Work out the finished part from the listing and answer in its coordinate system (mm). A direction names the side the tool comes from. Give positions to 0.01 mm unless a question says otherwise; leave off trailing zeros. Order: outer loops, then holes, each group sorted by start corner. A loop starts at its lowest first (then second) coordinate and runs counter-clockwise, first axis right, second up. Notation, with made-up numbers: (20.25, -26.5) -> (27.25, -26.5) arc R34 ccw to (27.25, 10.5) -> close; hole circle Ø6 at (52, -12.5). An arc over 180 degrees is marked (long way). Use a Markdown table: item, result. Add a question column.
```python
from build123d import *

# Parameters (mm, degrees)
BOSS_EXTRUDE1_DEPTH         = 10
CHAMFER1_SIZE               = 10
F_1_4_20_TAPPED_HOLE1_D     = 5.1054
F_1_4_20_TAPPED_HOLE1_DEPTH = 16.51


with BuildPart() as part:
    # Sketch1 → Boss-Extrude1 (new body)
    with BuildSketch(Plane.XY):
        with BuildLine():
            Line((0, -19.05), (0, 19.05))
            Line((0, 19.05), (25.4, 19.05))
            Line((25.4, 19.05), (30.82006403, 13.62993597))
            ThreePointArc((30.82006403, 13.62993597), (31.850108163, 12.941682484), (33.065128061, 12.7))
            Line((33.065128061, 12.7), (52.659871939, 12.7))
            ThreePointArc((52.659871939, 12.7), (53.874891837, 12.941682484), (54.90493597, 13.62993597))
            Line((54.90493597, 13.62993597), (60.325, 19.05))
            Line((60.325, 19.05), (73.025, 19.05))
            ThreePointArc((73.025, 19.05), (92.075, 0), (73.025, -19.05))
            Line((73.025, -19.05), (60.325, -19.05))
            Line((60.325, -19.05), (54.90493597, -13.62993597))
            ThreePointArc((54.90493597, -13.62993597), (53.874891837, -12.941682484), (52.659871939, -12.7))
            Line((52.659871939, -12.7), (33.065128061, -12.7))
            ThreePointArc((33.065128061, -12.7), (31.850108163, -12.941682484), (30.82006403, -13.62993597))
            Line((30.82006403, -13.62993597), (25.4, -19.05))
            Line((25.4, -19.05), (0, -19.05))
        make_face()
    extrude(amount=BOSS_EXTRUDE1_DEPTH)

    # Chamfer1
    chamfer1_edges = [part.edges().sort_by_distance(p)[0] for p in [
        (0, 0, 10),
    ]]
    chamfer(chamfer1_edges, length=CHAMFER1_SIZE - 0.0001)  # a hair under: the kernel refuses the full size

    # 1/4-20 Tapped Hole1
    with Locations(Plane(origin=(0, 0, 0), x_dir=(-1, 0, 0), z_dir=(0, 0, -1))):
        with Locations((-10, -9.144), (-10, 9.144)):
            Hole(F_1_4_20_TAPPED_HOLE1_D / 2, depth=F_1_4_20_TAPPED_HOLE1_DEPTH)

    # Sweep1: sweep along a path in Sketch8
    with BuildLine(Plane(origin=(0, 0, 0), x_dir=(1, 0, 0), z_dir=(0, 1, 0))) as sweep1_path:
        ThreePointArc((88.281159976, -10), (90.343330416, -73.5), (88.281159976, -137))
    # Sketch5 → Sweep1 (sweep)
    with BuildSketch(Plane.XY.offset(10)):
        with BuildLine():
            Line((89.202450062, -1.925597754), (89.202450062, 1.925597754))
            ThreePointArc((89.202450062, 1.925597754), (72.078047816, 19.05), (54.953645569, 1.925597754))
            Line((54.953645569, 1.925597754), (54.953645569, -1.925597754))
            ThreePointArc((54.953645569, -1.925597754), (72.078047816, -19.05), (89.202450062, -1.925597754))
        make_face()
    sweep(path=sweep1_path.line)


solid = part.part
```
1) Straight lines are drawn through the part: line 1 (Y direction, x = 10, z = 5); line 2 (Z direction, x = 32, y = 10); line 3 (Y direction, x = 62, z = 25). For each, find the intervals that lie inside material, in ascending order.
2) Flat-ended cylindrical pins translate along their axes: pin 1 (11 mm diameter, centred on x = 43.5, z = 4, fed in from +Y); pin 2 (1.5 mm diameter, centred on x = 15.5, y = 4.5, fed in from +Z); pin 3 (4 mm diameter, centred on x = 70.5, z = 60.5, fed in from -Y). Find the tip coordinate at first contact, or state that the pin passes through.
3) Which of the six approach directions +Z, -Z, +X, -X, +Y, -Y give full straight-line access (tool end or side, diameter ignored) to faces 1 (the flat face through (57.577, 16.302, 4.93)), 2 (the flat face through (43, -12.7, 5)), 3 (the flat face through (90, 0, 10))?
4) The part is cut by section A-A, the plane x = 48.5. Determine the outline of the cut face in (y, z), then the cut area to 3 significant figures.
5) Determine the mould class of faces 4 (the flat face through (5, 0, 5)), 5 (the flat face through (67, -19.05, 5)), 6 (the cylindrical face through (12.435, -8.377, 5.07)) for opening direction X: released by +X, released by -X, zero draft, split by the parting line, or undercut.
A:
| question | item | result |
|---|---|---|
| 1 | line 1 | -19.05 to -11.7, -6.59 to 6.59, 11.7 to 19.05 |
| 1 | line 2 | 0 to 10 |
| 1 | line 3 | -15.08 to 15.08 |
| 2 | pin 1 | y = 12.7 |
| 2 | pin 2 | z = 10 |
| 2 | pin 3 | y = -18.98 |
| 3 | face 1 | +Z, -Z, +Y |
| 3 | face 2 | +Z, -Z, -Y |
| 3 | face 3 | +X |
| 4 | outline | (-12.7, 0) -> (12.7, 0) -> (12.7, 10) -> (-12.7, 10) -> close |
| 4 | area | 254 mm^2 |
| 5 | face 4 | released by -X |
| 5 | face 5 | zero draft |
| 5 | face 6 | undercut |
